Work out the finished part from the listing and answer in its coordinate system (mm). Round coordinates to 2 decimals unless told otherwise and drop trailing zeros. Write each loop counter-clockwise with the first axis right and the second up, starting at its lowest first coordinate (ties: lowest second). Pieces come first, ordered by that corner, then holes. Notation, with made-up numbers: M 28,65 L 60,65 A16 cw 60,71 Z; hole C 80,31.5 d3. An arc over 180 degrees is marked long. One line per item, written item: value. Start each with the question number.
Q1. Given pin 1 Ø0.6 at (y, z) = (-0.5, 0.5) entering from -X, flat-ended and moving along its own axis, determine where the tip first touches the part or whether it passes through.
Q2. Find section B-B (x = 25.5). Write down the section's boundary in (y, z), and give its area (3 significant figures).
Q3. Consider probe 1 along X at (y, z) = (-4.5, 0.75); probe 2 along Y at (x, z) = (23, 0.7); probe 3 along X at (y, z) = (-19.5, 0.5). Determine where each line is inside the solid, lowest interval first.
Q4. Find section D-D (x = -20). Write down the section's boundary in (y, z).
Q5. Find section A-A (y = -32.5). Write down the section's boundary in (x, z).
Q6. Find section C-C (z = 0.9). Write down the section's boundary in (x, y).
from build123d import *

# Parameters (mm, degrees)
F0_R     = 1.5
F0_R_2   = 4.5
F1_DEPTH = 1.6


with BuildPart() as f1:
    # F0 (on Top) → F1 (new body)
    with BuildSketch(Plane.XY):
        with BuildLine():
            Line((31.234043, -8.719558), (31.234043, -1.418333))
            ThreePointArc((31.234043, -1.418333), (29.769577, 2.117201), (26.234043, 3.581667))
            Line((26.234043, 3.581667), (1.948889, 3.581667))
            ThreePointArc((1.948889, 3.581667), (-0.879538, 2.410094), (-2.051111, -0.418333))
            Line((-2.051111, -0.418333), (-2.051111, -0.933739))
            ThreePointArc((-2.051111, -0.933739), (-2.84194, -3.321461), (-4.90172, -4.765044))
            Line((-4.90172, -4.765044), (-29.545943, -12.158312))
            ThreePointArc((-29.545943, -12.158312), (-31.605723, -13.601895), (-32.396551, -15.989617))
            Line((-32.396551, -15.989617), (-32.396551, -20.383074))
            ThreePointArc((-32.396551, -20.383074), (-31.572894, -22.814297), (-29.441127, -24.244273))
            Line((-29.441127, -24.244273), (5.201511, -33.616194))
            ThreePointArc((5.201511, -33.616194), (6.642545, -34.343427), (7.678821, -35.580996))
            Line((7.678821, -35.580996), (8.385379, -36.893176))
            ThreePointArc((8.385379, -36.893176), (9.856117, -38.430843), (11.907264, -38.996778))
            Line((11.907264, -38.996778), (15.831667, -38.996778))
            ThreePointArc((15.831667, -38.996778), (18.619917, -38.14716), (20.460587, -35.887045))
            Line((20.460587, -35.887045), (30.937178, -10.231771))
            ThreePointArc((30.937178, -10.231771), (31.159125, -9.490096), (31.234043, -8.719558))
        make_face()
        with Locations((-29.198352, -18.399177)):
            Circle(F0_R, mode=Mode.SUBTRACT)
        with Locations((-8.879622, -17.901169)):
            Circle(F0_R, mode=Mode.SUBTRACT)
        with Locations((14.315047, -31.251039)):
            Circle(F0_R_2, mode=Mode.SUBTRACT)
        with Locations((5.875676, -4.47092)):
            Circle(F0_R_2, mode=Mode.SUBTRACT)
        with Locations((23.163911, -4.47092)):
            Circle(F0_R_2, mode=Mode.SUBTRACT)
    extrude(amount=F1_DEPTH)


solid = f1.part
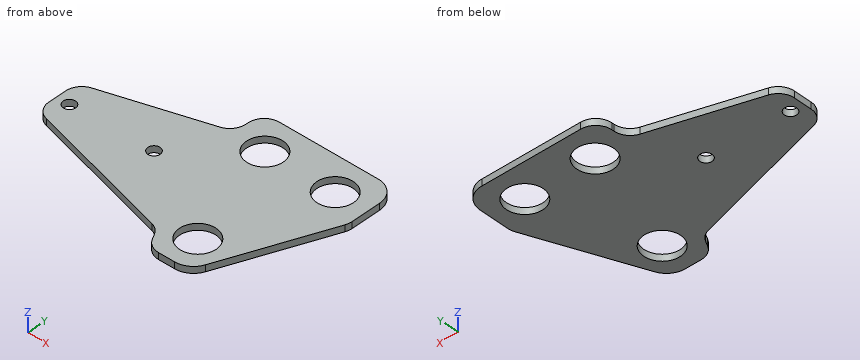
The answers:
1. pin 1: x = -2.05
2. outline: M -23.55,0 L -8.32,0 L -8.32,1.6 L -23.55,1.6 Z; M -0.62,0 L 3.58,0 L 3.58,1.6 L -0.62,1.6 Z
2. area: 31.1 mm2
3. probe 1: -4.24 to 1.38, 10.38 to 18.66, 27.66 to 31.23
3. probe 2: -29.67 to -8.97, 0.03 to 3.58
3. probe 3: -32.4 to -30.22, -28.18 to 27.15
4. outline: M -26.8,0 L -9.29,0 L -9.29,1.6 L -26.8,1.6 Z
5. outline: M 1.08,0 L 9.99,0 L 9.99,1.6 L 1.08,1.6 Z; M 18.64,0 L 21.84,0 L 21.84,1.6 L 18.64,1.6 Z
6. outline: M -32.4,-20.38 A4 ccw -29.44,-24.24 L 5.2,-33.62 A4 cw 7.68,-35.58 L 8.39,-36.89 A4 ccw 11.91,-39 L 15.83,-39 A5 ccw 20.46,-35.89 L 30.94,-10.23 A4 ccw 31.23,-8.72 L 31.23,-1.42 A5 ccw 26.23,3.58 L 1.95,3.58 A4 ccw -2.05,-0.42 L -2.05,-0.93 A4 cw -4.9,-4.77 L -29.55,-12.16 A4 ccw -32.4,-15.99 Z; hole C -29.2,-18.4 d3; hole C -8.88,-17.9 d3; hole C 5.88,-4.47 d9; hole C 14.32,-31.25 d9; hole C 23.16,-4.47 d9
